Input: part model. Units: mm. Frame: model coordinates. A direction names the side the tool comes from. Give positions to 0.01 mm unless a question says otherwise; leave off trailing zeros. Order: outer loops, then holes, each group sorted by start corner. A loop starts at its lowest first (then second) coordinate and runs counter-clockwise, first axis right, second up. Notation, with made-up numbers: (-18, -39.75) - (-1, -39.75) arc R22 ccw to (-1, -12.75) - close; hole circle Ø1 at (-33.75, -31.75). An arc over 180 degrees is marked (long way). Answer in a Markdown table with one row per item. Add a question column.
Autodesk Inventor part; units mm, degrees
ref_plane "YZ Plane" through (0, 0, 0) normal (1, 0, 0) x (0, 1, 0)
ref_plane "XZ Plane" through (0, 0, 0) normal (0, 1, 0) x (-1, 0, 0)
ref_plane "XY Plane" through (0, 0, 0) normal (0, 0, 1) x (1, 0, 0)
sketch "Szkic1" plane through (0, 0, 0) normal (0, 0, 1) x (1, 0, 0)
  circle A0 centre (0, 0) radius 18
  dimension "d0" = 36
extrude "Wyciągnięcie proste1" add sketch "Szkic1" along normal blind 2
sketch "Szkic2" plane through (0, 0, 2) normal (0, 0, 1) x (1, 0, 0)
  circle A0 centre (0, 0) radius 1.5
  line L0 (0, 25.2) -> (0, -25.2)
  line L1 (-25.2, 0) -> (25.2, 0)
  line L2 (-1.118, 1) -> (1.118, 1)
  circle A1 centre (0, 0) radius 18
  dimension "d3" = 3
  dimension "d4" = 1
extrude "Wyciągnięcie proste2" add sketch "Szkic2" along normal blind 4 contours L1 L0 L2 A0 | A0 L0 L1 | A0 L1 L0 | L1 A0 L2 L0
sketch "Szkic3" plane through (0, 0, 2) normal (0, 0, 1) x (1, 0, 0)
  line L0 (-1.118, 1) -> (1.118, 1)
  arc A0 (-1.118, 1) -> (1.118, 1) centre (0, 0) ccw
  circle A1 centre (0, 0) radius 18
  circle A2 centre (0, 0) radius 16.1
  dimension "d8" = 32.2
extrude "Wyciągnięcie proste3" add sketch "Szkic3" along normal blind 8 contours A1
properties part number "forma_do_kół"
Q1. Section B-B, the plane y = 0. Return loops of the section in (x, z).
Q2. Pull-direction query (Y, two-part tool) for faces 1 (the flat face through (-13.4, -9.2, 10)), 2 (the cylindrical face through (0, -1.5, 4)), 3 (the cylindrical face through (-2.343, -17.847, 4.93)); classes: +Y half, -Y half, draft (parallel to the pull), parting line (faces both ways), or undercut.
Q3. Section C-C, the plane x = 9. Return loops of the section in (y, z), then the cut area to 3 significant figures.
Q4. Section D-D, the plane y = -15. Return loops of the section in (x, z).
Q5. Access query for faces 4 (the flat face through (0, 0, 0)), 5 (the flat face through (0, 0, 6)). Directions: +Z, -Z, +X, -X, +Y, -Y. A direction counts if a zero-diameter tool reaches every point of the face in a straight line with its end or side. Return the directions, or none.
Q6. Section A-A, the plane x = 0. Return loops of the section in (y, z).
Q7. Contact query for flat-ended pins moving along their axis: P1, Ø3, axis at x = -6, z = 8.5, coming from the +Y side; P2, Ø2, axis at x = -2, y = 12.5, coming from the +Z side; P3, Ø3, axis at x = 0, y = -0.5, coming from the +Z side. Output: stop coordinate, or through.
Q8. Line query: probe 1 along Y at (x, z) = (0, 5.75); probe 2 along Y at (x, z) = (0, 7.25); probe 3 along Z at (x, y) = (2.5, -13.5). Output: solid intervals per line, ascending.
Computed:
| question | item | result |
|---|---|---|
| 1 | outline | (-18, 0) - (18, 0) - (18, 10) - (16.1, 10) - (16.1, 2) - (1.5, 2) - (1.5, 6) - (-1.5, 6) - (-1.5, 2) - (-16.1, 2) - (-16.1, 10) - (-18, 10) - close |
| 2 | face 1 | draft |
| 2 | face 2 | undercut |
| 2 | face 3 | parting line |
| 3 | outline | (-15.59, 0) - (15.59, 0) - (15.59, 10) - (13.35, 10) - (13.35, 2) - (-13.35, 2) - (-13.35, 10) - (-15.59, 10) - close |
| 3 | area | 98.2 mm^2 |
| 4 | outline | (-9.95, 0) - (9.95, 0) - (9.95, 10) - (5.85, 10) - (5.85, 2) - (-5.85, 2) - (-5.85, 10) - (-9.95, 10) - close |
| 5 | face 4 | -Z, +X, -X, +Y, -Y |
| 5 | face 5 | +Z |
| 6 | outline | (-18, 0) - (18, 0) - (18, 10) - (16.1, 10) - (16.1, 2) - (1, 2) - (1, 6) - (-1.5, 6) - (-1.5, 2) - (-16.1, 2) - (-16.1, 10) - (-18, 10) - close |
| 7 | P1 | stops at y = 17.43 |
| 7 | P2 | stops at z = 2 |
| 7 | P3 | stops at z = 6 |
| 8 | probe 1 | y = -18 to -16.1, -1.5 to 1, 16.1 to 18 |
| 8 | probe 2 | y = -18 to -16.1, 16.1 to 18 |
| 8 | probe 3 | z = 0 to 2 |
